Here's how the part is built. I have some questions about the finished solid (model axes, mm). Round coordinates to 2 decimals unless told otherwise and drop trailing zeros. Write each loop counter-clockwise with the first axis right and the second up, starting at its lowest first coordinate (ties: lowest second). Pieces come first, ordered by that corner, then holes. Notation, with made-up numbers: (78.25, 64) -> (119.25, 64) arc R17 cw to (119.25, 80) -> close; hole circle Ø10 at (-13, 40.25). An arc over 180 degrees is marked (long way). Put each result on its own line as item: value. Start each with the question number.
1. For pin 1 (4 mm diameter, centred on x = -4.06, z = -46, fed in from -Y); pin 2 (1.5 mm diameter, centred on y = 10.5, z = -37.5, fed in from -X); pin 3 (8 mm diameter, centred on x = 6.5, z = -14, fed in from +Y); pin 4 (5 mm diameter, centred on x = -2.5, z = 11.5, fed in from +Y), each with a flat end and sliding along its axis, tell me the tip position at first contact or that it passes through.
2. Suppose I cut it at B-B (z = 46). Count the separate pieces of the cut face and the enclosed holes in it, then the cut area to 3 significant figures.
3. Suppose I cut it at C-C (x = 6.25). Please give me the cut outline in (y, z), then the cut area to 3 significant figures.
4. I need wall thicknesses on probe 1 along X at (y, z) = (3.5, 38) (1 decimal); probe 2 along Y at (x, z) = (8.25, -46); probe 3 along Y at (x, z) = (8.15, 46). Which ranges of each line are inside material? Lowest first, please. Write a range as from..to.
```python
from build123d import *

# Parameters (mm, degrees)
BOSS_EXTRUDE1_DEPTH                               = 50
CSK_FOR_4_FLAT_HEAD_MACHINE_SCREW_100_D           = 3.2639
CSK_FOR_4_FLAT_HEAD_MACHINE_SCREW_100_CSINK_D     = 5.715
CSK_FOR_4_FLAT_HEAD_MACHINE_SCREW_100_CSINK_ANGLE = 100
CSK_FOR_4_FLAT_HEAD_MACHINE_SCREW_2_D             = 3.2639
CSK_FOR_4_FLAT_HEAD_MACHINE_SCREW_2_CSINK_D       = 5.715
CSK_FOR_4_FLAT_HEAD_MACHINE_SCREW_2_CSINK_ANGLE   = 100
FILLET1_R                                         = 1
CUT_EXTRUDE1_DEPTH                                = 25


with BuildPart() as part:
    # Sketch2 → Boss-Extrude1 (new, symmetric)
    with BuildSketch(Plane.XY):
        with BuildLine():
            Line((-9.525, 0), (9.525, 0))
            Line((9.525, 0), (9.525, 19.05))
            Line((9.525, 19.05), (8.73125, 19.05))
            ThreePointArc((8.73125, 19.05), (8.169983992, 18.817516008), (7.9375, 18.25625))
            Line((7.9375, 18.25625), (7.9375, 2.38125))
            ThreePointArc((7.9375, 2.38125), (7.705016008, 1.819983992), (7.14375, 1.5875))
            Line((7.14375, 1.5875), (-8.73125, 1.5875))
            ThreePointArc((-8.73125, 1.5875), (-9.292516008, 1.355016008), (-9.525, 0.79375))
            Line((-9.525, 0.79375), (-9.525, 0))
        make_face()
    extrude(amount=BOSS_EXTRUDE1_DEPTH, both=True)

    # CSK for _4 Flat Head Machine Screw _100 (through all)
    with Locations(Plane(origin=(0, 0, 0), x_dir=(-1, 0, 0), z_dir=(0, -1, 0))):
        with Locations((4.0625, -46), (4.0625, 46)):
            CounterSinkHole(CSK_FOR_4_FLAT_HEAD_MACHINE_SCREW_100_D / 2, CSK_FOR_4_FLAT_HEAD_MACHINE_SCREW_100_CSINK_D / 2, counter_sink_angle=CSK_FOR_4_FLAT_HEAD_MACHINE_SCREW_100_CSINK_ANGLE)

    # CSK for _4 Flat Head Machine Screw _ 2 (through all)
    with Locations(Plane(origin=(9.525, 0, 0), x_dir=(0, 0, -1), z_dir=(1, 0, 0))):
        with Locations((-46, 13.5875), (46, 13.5875)):
            CounterSinkHole(CSK_FOR_4_FLAT_HEAD_MACHINE_SCREW_2_D / 2, CSK_FOR_4_FLAT_HEAD_MACHINE_SCREW_2_CSINK_D / 2, counter_sink_angle=CSK_FOR_4_FLAT_HEAD_MACHINE_SCREW_2_CSINK_ANGLE)

    # Fillet1
    fillet1_edges = [part.edges().sort_by_distance(p)[0] for p in [
        (9.525, 0, 0),
    ]]
    fillet(fillet1_edges, radius=FILLET1_R)

    # Sketch24 → Cut-Extrude1 (cut)
    with BuildSketch(Plane.XY.offset(50)):
        Polygon((2.9375, 1.5875), (7.9375, 6.5875), (7.9375, 1.5875), align=None)
    cut_extrude1 = extrude(amount=-CUT_EXTRUDE1_DEPTH, mode=Mode.SUBTRACT)

    # Mirror1: Cut-Extrude1 across plane
    add(cut_extrude1.mirror(Plane.XY), mode=Mode.SUBTRACT)


solid = part.part
```
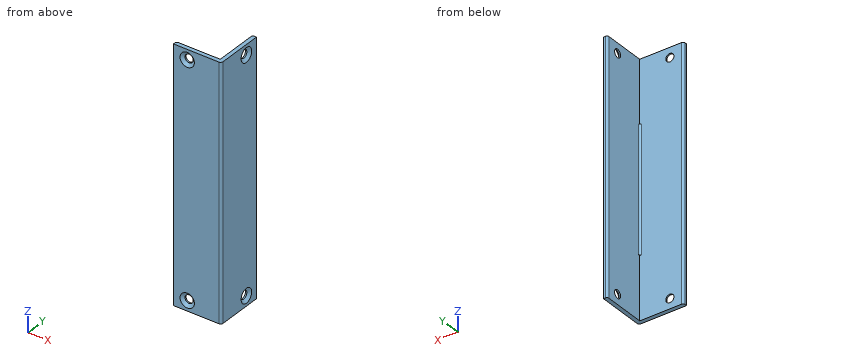
Verdict:
1. pin 1: stops at y = 0.72
1. pin 2: stops at x = 7.94
1. pin 3: stops at y = 19.05
1. pin 4: stops at y = 1.59
2. separate pieces: 3
2. enclosed holes: 0
2. area: 44.6 mm^2
3. outline: (0, -50) -> (1.59, -50) -> (1.59, 50) -> (0, 50) -> close
3. area: 159 mm^2
4. probe 1: x = 7.9..9.5
4. probe 2: y = 0..11.96, 15.22..18.89
4. probe 3: y = 0..11.96, 15.22..18.8
